Part model, mm, in its own coordinate system. Face numbers are marked on the shaded views. Coordinates: 2 decimals unless noted, no trailing zeros. Order: outer loops, then holes, each group sorted by start corner. A loop starts at its lowest first (then second) coordinate and runs counter-clockwise, first axis right, second up. Notation, with made-up numbers: (22, 41.5) - (47, 41.5) arc R16 cw to (47, 70.5) - close; hole circle Ø4 at (33.25, 36). An arc over 180 degrees is marked (long way). Use a Markdown table: item, result. Add a question column.
1) Wall check: L1, parallel to Z at x = 1, y = 0.5 (3 decimals); L2, parallel to X at y = 0.35, z = 0.75 (3 decimals); L3, parallel to X at y = 0.15, z = 0.5 (3 decimals). Give the ranges that are in metal, low to high. Write a range as [from, to].
2) Saw through at D-D on z = -1.75. List the corners of the cut face in (x, y) (3 decimals), then the cut area to 3 significant figures.
3) Saw through at B-B on y = 0.2. List the corners of the cut face in (x, z) (3 decimals), then the cut area to 3 significant figures.
4) Two-plate mould, pull along X, no slides. Class the marked faces 1, 2 and 3: +X half, -X half, draft (parallel to the pull), parting line (faces both ways), or undercut.
5) Saw through at A-A on z = 0. List the corners of the cut face in (x, y) (3 decimals), then the cut area to 3 significant figures.
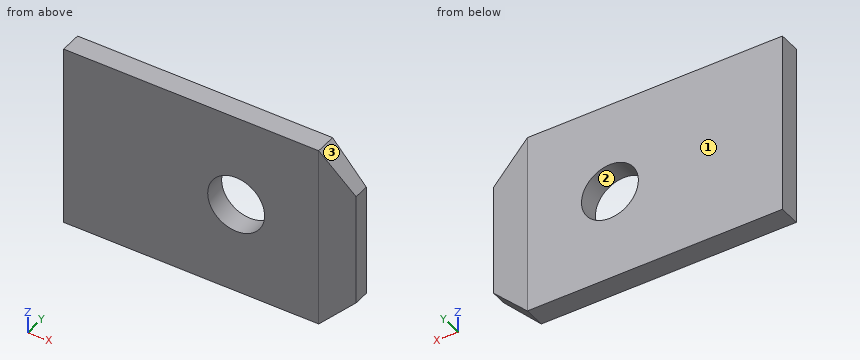
Autodesk Inventor part; units mm, degrees
ref_plane "YZ Plane" through (0, 0, 0) normal (1, 0, 0) x (0, 1, 0)
ref_plane "XZ Plane" through (0, 0, 0) normal (0, 1, 0) x (-1, 0, 0)
ref_plane "XY Plane" through (0, 0, 0) normal (0, 0, 1) x (1, 0, 0)
sketch "Sketch1" plane through (0, 0, 0) normal (0, 1, 0) x (-1, 0, 0)
  line L0 (5.105, 3.225) -> (-3.855, 3.225)
  line L1 (-5.105, 1.975) -> (-5.105, -1.975)
  line L2 (-3.855, -3.225) -> (5.105, -3.225)
  line L3 (5.105, -3.225) -> (5.105, 3.225)
  line L4 (5.105, 0) -> (-5.105, 0) construction
  line L5 (-3.855, 3.225) -> (-5.105, 1.975)
  line L6 (-5.105, -1.975) -> (-3.855, -3.225)
  line L7 (-4.48, 2.6) -> (-1.88, 0) construction
  line L8 (-4.48, -2.6) -> (-1.88, 0) construction
  circle A0 centre (-0.955, 0) radius 1
  point P0 (0, 0)
  point P1 (0, 0)
  dimension "d0" = 6.45
  dimension "d1" = 10.21
  dimension "d2" = 1.25
  dimension "d3" = 2
  dimension "d4" = 3.15
extrude "Extrusion1" add sketch "Sketch1" along normal blind 0.75
chamfer "Chamfer1" distance 1.25 distance2 0.1 1 edges at (5.105, 0.75, 0) measured on face at (-3.4183, 0.75, 0)
chamfer "Chamfer2" distance 0.1 distance2 1.25 1 edges at (5.105, 0, 0) measured on face at (5.105, 0.2167, 0.6583)
properties part number "Toggle_Pin_Brass" material "Brass, Soft Yellow"
Results are:
| question | item | result |
|---|---|---|
| 1 | L1 | [-3.225, -0.999], [0.999, 3.225] |
| 1 | L2 | [-5.105, 0.294], [1.616, 5.105] |
| 1 | L3 | [-5.105, 0.089], [1.821, 5.105] |
| 2 | outline | (-5.105, 0) - (3.855, 0) - (5.105, 0.1) - (5.105, 0.65) - (3.855, 0.75) - (-5.105, 0.75) - close |
| 2 | area | 7.53 mm2 |
| 3 | outline | (-5.105, -3.225) - (3.855, -3.225) - (5.105, -1.975) - (5.105, 1.975) - (3.855, 3.225) - (-5.105, 3.225) - close; hole circle Ø2 at (0.955, 0) |
| 3 | area | 61.2 mm2 |
| 4 | face 1 | draft |
| 4 | face 2 | undercut |
| 4 | face 3 | +X half |
| 5 | outline | (-5.105, 0) - (-0.045, 0) - (-0.045, 0.75) - (-5.105, 0.75) - close; (1.955, 0) - (3.855, 0) - (5.105, 0.1) - (5.105, 0.65) - (3.855, 0.75) - (1.955, 0.75) - close |
| 5 | area | 6.03 mm2 |
